Here's how the part is built. I have some questions about the finished solid (model axes, mm). Face numbers are marked on the shaded views. A direction names the side the tool comes from. Round coordinates to 2 decimals unless told otherwise and drop trailing zeros. Write each loop counter-clockwise with the first axis right and the second up, starting at its lowest first coordinate (ties: lowest second). Pieces come first, ordered by that corner, then holes. Notation, with made-up numbers: (59, 85) - (64, 85) arc R28 ccw to (64, 112) - close; hole circle Ø1 at (14.5, -30). An arc over 180 degrees is marked (long way). Use one line per item in the form item = value. Start each with the question number.
1. Which directions (+Z, -Z, +X, -X, +Y, -Y) give clear straight access to the entire face, cutting with the end or side of a thin tool? Please do the marked faces 1, 2 and 3.
2. Will these pins go through, and if not, where does the flat tip stop? pin 1 (4 mm diameter, centred on x = -338, z = -46, fed in from +Y); pin 2 (1 mm diameter, centred on y = 302.5, z = -30, fed in from -X); pin 3 (10 mm diameter, centred on x = -159, z = -60, fed in from -Y).
3. I want a section at B-B, the plane y = -492. List the corners of the cut face in (x, z) for me (3 decimals).
4. I want a section at A-A, the plane y = 0. List the corners of the cut face in (x, z) for me, plus the area to 3 significant figures.
5. We'd pull the mould along Y, two halves only. Please class the marked faces 4, 5 and 6: +Y half, -Y half, draft (parallel to the pull), parting line (faces both ways), or undercut.
6. If I drill on line 1 along Y through (x, z) = (0, -40); line 2 along X through (y, z) = (-315, 39); line 3 along Y through (x, z) = (68.5, -53), over which ranges is the centre line in solid material (lowest first)?
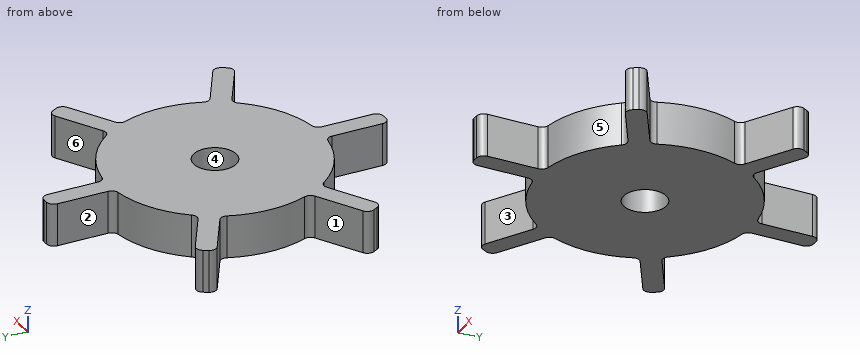
```python
from build123d import *

# Parameters (mm, degrees)
SKETCH1_R                = 381
SKETCH1_R_2              = 76.2
BOSS_EXTRUDE1_DEPTH      = 76.2
BOSS_EXTRUDE2_DEPTH      = 152.4
FILLET1_R                = 25.4
CIRPATTERN1_COUNT        = 6
FILLET1_OF_CIRPATTERN1_R = 25.4


with BuildPart() as part:
    # Sketch1 → Boss-Extrude1 (new, symmetric)
    with BuildSketch(Plane.XY):
        with Locations(Location((0, 0, 0), (0, 0, 180))):
            Circle(SKETCH1_R)
        with Locations(Location((0, 0, 0), (0, 0, 180))):
            Circle(SKETCH1_R_2, mode=Mode.SUBTRACT)
    extrude(amount=BOSS_EXTRUDE1_DEPTH, both=True)

    # Sketch2 → Boss-Extrude2 (add)
    with BuildSketch(Plane.XY.offset(76.2)):
        with BuildLine():
            Line((-34.925, 379.395893988), (-34.925, 609.6))
            Line((-34.925, 609.6), (34.925, 609.6))
            Line((34.925, 609.6), (34.925, 379.395893988))
            ThreePointArc((34.925, 379.395893988), (0, 381), (-34.925, 379.395893988))
        make_face()
    boss_extrude2 = extrude(amount=-BOSS_EXTRUDE2_DEPTH)

    # Fillet1
    fillet1_edges = [part.edges().sort_by_distance(p)[0] for p in [
        (34.925, 379.395893988, 0),
        (-34.925, 379.395893988, 0),
        (-34.925, 609.6, 0),
        (34.925, 609.6, 0),
    ]]
    fillet(fillet1_edges, radius=FILLET1_R)

    # CirPattern1: Boss-Extrude2 ×6 about axis
    cirpattern1_axis = Axis((0, 0, 0), (0, 0, 1))
    for i in range(1, CIRPATTERN1_COUNT):
        add(boss_extrude2.rotate(cirpattern1_axis, i * 360 / CIRPATTERN1_COUNT))

    # Fillet1 of CirPattern1
    fillet1_of_cirpattern1_edges = [part.edges().sort_by_distance(p)[0] for p in [
        (-311.103982285, 219.943884221, 0),
        (-346.028982285, 159.452009767, 0),
        (-545.391586147, 274.554062773, 0),
        (-510.466586147, 335.045937227, 0),
        (-346.028982285, -159.452009767, 0),
        (-311.103982285, -219.943884221, 0),
        (-510.466586147, -335.045937227, 0),
        (-545.391586147, -274.554062773, 0),
        (-34.925, -379.395893988, 0),
        (34.925, -379.395893988, 0),
        (34.925, -609.6, 0),
        (-34.925, -609.6, 0),
        (311.103982285, -219.943884221, 0),
        (346.028982285, -159.452009767, 0),
        (545.391586147, -274.554062773, 0),
        (510.466586147, -335.045937227, 0),
        (346.028982285, 159.452009767, 0),
        (311.103982285, 219.943884221, 0),
        (510.466586147, 335.045937227, 0),
        (545.391586147, 274.554062773, 0),
    ]]
    fillet(fillet1_of_cirpattern1_edges, radius=FILLET1_OF_CIRPATTERN1_R)


solid = part.part
```
Model answer:
q1.face_1 = +Z, -Z, -X
q1.face_2 = +Z, -Z, -X, +Y
q1.face_3 = +Z, -Z, -Y
q2.pin_1 = 236.63
q2.pin_2 = -529.55
q2.pin_3 = -348.49
q3.outline = (-34.925, -76.2) - (34.925, -76.2) - (34.925, 76.2) - (-34.925, 76.2) - close
q4.outline = (-381, -76.2) - (-76.2, -76.2) - (-76.2, 76.2) - (-381, 76.2) - close; (76.2, -76.2) - (381, -76.2) - (381, 76.2) - (76.2, 76.2) - close
q4.area = 92,900 mm2
q5.face_4 = undercut
q5.face_5 = -Y half
q5.face_6 = +Y half
q6.line_1 = -609.6 to -76.2, 76.2 to 609.6
q6.line_2 = -521.92 to -475.75, -214.33 to 214.33, 475.75 to 521.92
q6.line_3 = -374.79 to -33.38, 33.38 to 374.79
